Source: CAD feature listing. Evaluate the final solid. Frame: model axes, mm. Give positions to 0.01 mm unless a question says otherwise; leave off trailing zeros. Order: outer loops, then holes, each group sorted by start corner. A loop starts at its lowest first (then second) coordinate and runs counter-clockwise, first axis right, second up. Notation, with made-up numbers: (7, 29.25) -> (66, 29.25) arc R14 cw to (66, 50.25) -> close; hole circle Ø6 at (54, 67.25). An arc over 180 degrees is marked (long way). Answer in a Markdown table with one row per item.
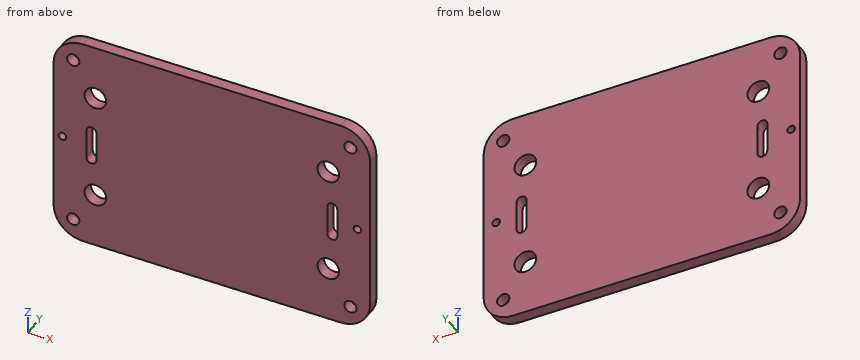
```python
from build123d import *

# Parameters (mm, degrees)
SCHIZZO1_R                   = 2.1
SCHIZZO1_R_2                 = 3.7
SCHIZZO1_R_3                 = 1.3
ESTRUSIONE_ESTRUSIONE1_DEPTH = 4


with BuildPart() as part:
    # Schizzo1 → Estrusione-Estrusione1 (new body)
    with BuildSketch(Plane(origin=(0, 0, 0), x_dir=(1, 0, 0), z_dir=(0, 1, 0))):
        with BuildLine():
            Line((-10.05, 0), (-98.05, 0))
            ThreePointArc((-98.05, 0), (-105.156423151, 2.943576849), (-108.1, 10.05))
            Line((-108.1, 10.05), (-108.1, 62.95))
            ThreePointArc((-108.1, 62.95), (-105.156423151, 70.056423151), (-98.05, 73))
            Line((-98.05, 73), (-10.05, 73))
            ThreePointArc((-10.05, 73), (-2.943576849, 70.056423151), (0, 62.95))
            Line((0, 62.95), (0, 10.05))
            ThreePointArc((0, 10.05), (-2.943576849, 2.943576849), (-10.05, 0))
        make_face()
        with Locations(Location((-6.7, 66, 0), (0, 0, 270))):
            Circle(SCHIZZO1_R, mode=Mode.SUBTRACT)
        with Locations(Location((-6.7, 7, 0), (0, 0, 270))):
            Circle(SCHIZZO1_R, mode=Mode.SUBTRACT)
        with Locations(Location((-101.4, 66, 0), (0, 0, 270))):
            Circle(SCHIZZO1_R, mode=Mode.SUBTRACT)
        with Locations(Location((-101.4, 7, 0), (0, 0, 270))):
            Circle(SCHIZZO1_R, mode=Mode.SUBTRACT)
        with Locations(Location((-93.85, 54.45, 0), (0, 0, 270))):
            Circle(SCHIZZO1_R_2, mode=Mode.SUBTRACT)
        with Locations(Location((-93.85, 18.55, 0), (0, 0, 270))):
            Circle(SCHIZZO1_R_2, mode=Mode.SUBTRACT)
        with Locations(Location((-14.25, 18.55, 0), (0, 0, 270))):
            Circle(SCHIZZO1_R_2, mode=Mode.SUBTRACT)
        with Locations(Location((-14.25, 54.45, 0), (0, 0, 270))):
            Circle(SCHIZZO1_R_2, mode=Mode.SUBTRACT)
        with Locations(Location((-4.3, 36.5, 0), (0, 0, 270))):
            Circle(SCHIZZO1_R_3, mode=Mode.SUBTRACT)
        with Locations(Location((-105.1, 36.5, 0), (0, 0, 270))):
            Circle(SCHIZZO1_R_3, mode=Mode.SUBTRACT)
        with BuildLine():
            Line((-96.9, 31.5), (-96.9, 41.5))
            ThreePointArc((-96.9, 41.5), (-95.2, 43.2), (-93.5, 41.5))
            Line((-93.5, 41.5), (-93.5, 31.5))
            ThreePointArc((-93.5, 31.5), (-95.2, 29.8), (-96.9, 31.5))
        make_face(mode=Mode.SUBTRACT)
        with BuildLine():
            Line((-14.6, 31.5), (-14.6, 41.5))
            ThreePointArc((-14.6, 41.5), (-12.9, 43.2), (-11.2, 41.5))
            Line((-11.2, 41.5), (-11.2, 31.5))
            ThreePointArc((-11.2, 31.5), (-12.9, 29.8), (-14.6, 31.5))
        make_face(mode=Mode.SUBTRACT)
    extrude(amount=ESTRUSIONE_ESTRUSIONE1_DEPTH)


solid = part.part
```
(1) Section query D-D (x = -6.7). Return the cut outline in (y, z).
A:
| item | result |
|---|---|
| outline | (0, -72.43) -> (4, -72.43) -> (4, -68.1) -> (0, -68.1) -> close; (0, -63.9) -> (4, -63.9) -> (4, -9.1) -> (0, -9.1) -> close; (0, -4.9) -> (4, -4.9) -> (4, -0.57) -> (0, -0.57) -> close |
(2) Section query C-C (x = -95.2). Return the cut outline in (y, z), plus the area to 3 significant figures.
A:
| item | result |
|---|---|
| outline | (0, -73) -> (4, -73) -> (4, -57.89) -> (0, -57.89) -> close; (0, -51.01) -> (4, -51.01) -> (4, -43.2) -> (0, -43.2) -> close; (0, -29.8) -> (4, -29.8) -> (4, -21.99) -> (0, -21.99) -> close; (0, -15.11) -> (4, -15.11) -> (4, 0) -> (0, 0) -> close |
| area | 183 mm^2 |
(3) First-contact query: pin 1 Ø8.5 at (x, z) = (-93.85, -18.55) entering from -Y. Flat tip, straight axial feed; report the tip coordinate or a pass-through.
A:
| item | result |
|---|---|
| pin 1 | stops at y = 0 |
(4) Section query B-B (y = 1.4). Give the number of separate pieces and of enclosed holes in the cut face, plus the area to 3 significant figures.
A:
| item | result |
|---|---|
| separate pieces | 1 |
| enclosed holes | 12 |
| area | 7,480 mm^2 |
(5) Section query A-A (z = -54.45). Return the cut outline in (x, y).
A:
| item | result |
|---|---|
| outline | (-108.1, 0) -> (-97.55, 0) -> (-97.55, 4) -> (-108.1, 4) -> close; (-90.15, 0) -> (-17.95, 0) -> (-17.95, 4) -> (-90.15, 4) -> close; (-10.55, 0) -> (0, 0) -> (0, 4) -> (-10.55, 4) -> close |
(6) Ray query, probe 1 along X at (y, z) = (2.8, -36.5); probe 2 along X at (y, z) = (2.7, -54.45); probe 3 along X at (y, z) = (1.35, -7). Return the intervals inside material, ascending.
A:
| item | result |
|---|---|
| probe 1 | x = -108.1 to -106.4, -103.8 to -96.9, -93.5 to -14.6, -11.2 to -5.6, -3 to 0 |
| probe 2 | x = -108.1 to -97.55, -90.15 to -17.95, -10.55 to 0 |
| probe 3 | x = -107.63 to -103.5, -99.3 to -8.8, -4.6 to -0.47 |
